Geometry: final body of the model. Coordinates: model frame, mm. Face numbers are marked on the shaded views. A direction names the side the tool comes from. Coordinates: 2 decimals unless noted, no trailing zeros. Write each loop counter-clockwise with the first axis right and the second up, starting at its lowest first coordinate (ties: lowest second). Pieces come first, ordered by that corner, then holes. Notation, with made-up numbers: (17.25, 42.5) - (67.25, 42.5) arc R34 cw to (67.25, 77.5) - close; hole circle Ø4 at (22.5, 34). An arc over 180 degrees is marked (long way). Answer as a JSON object with one key per item and string values. Group by question number.
Item 1: Mould query, pull axis Y, two halves, no side actions, for the marked faces 1, 2 and 3. Classes: pulls with the +Y half, pulls with the -Y half, needs draft (parallel to the pull), parting line crosses it, or undercut.
Item 2: Section B-B on x = 0. Return loops of the section in (y, z), and give its area (3 significant figures).
Item 3: Section A-A on y = 0. Return loops of the section in (x, z), and give its area (3 significant figures).
Item 4: Section D-D on y = 2.2. Return loops of the section in (x, z).
Item 5: Set-up query: the marked faces 4, 5 and 6. Return all of +Z, -Z, +X, -X, +Y, -Y with unobstructed straight access to the full face (end or side cutting, diameter ignored); none if empty.
Item 6: Line query: line 1 along Y through (x, z) = (0, -4.25); line 2 along X through (y, z) = (0, -4); line 3 along Y through (x, z) = (0, 0.5). Output: solid intervals per line, ascending. Write a range as from..to.
Item 7: Section C-C on z = 0. Return loops of the section in (x, y), and give its area (3 significant figures).
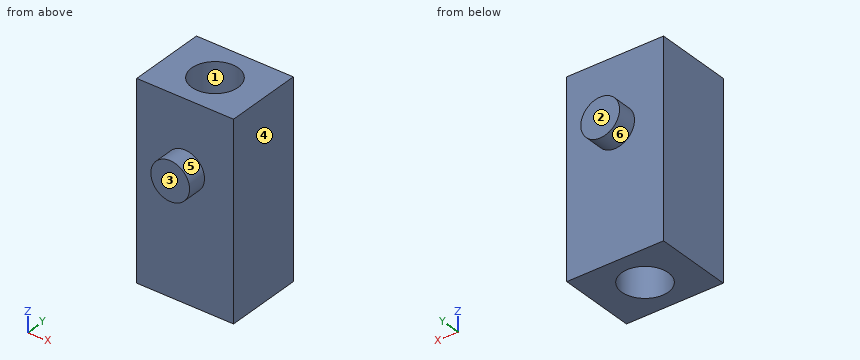
Autodesk Inventor part; units mm, degrees
ref_plane "YZ Plane" through (0, 0, 0) normal (1, 0, 0) x (0, 1, 0)
ref_plane "XZ Plane" through (0, 0, 0) normal (0, 1, 0) x (-1, 0, 0)
ref_plane "XY Plane" through (0, 0, 0) normal (0, 0, 1) x (1, 0, 0)
sketch "スケッチ1" plane through (0, 0, 0) normal (0, 1, 0) x (-1, 0, 0)
  line L0 (2.5, 3.5) -> (-2.5, 3.5)
  line L1 (-2.5, 3.5) -> (-2.5, -6.5)
  line L2 (-2.5, -6.5) -> (2.5, -6.5)
  line L3 (2.5, -6.5) -> (2.5, 3.5)
  point P0 (0, 0)
  point P1 (0, 3.5)
  dimension "d0" = 5
  dimension "d15" = 10
  dimension "d46" = 3.5
extrude "押し出し1" add sketch "スケッチ1" along normal mid plane 4
sketch "スケッチ2" plane through (0, 0, 0) normal (0, 1, 0) x (-1, 0, 0)
  circle A0 centre (0, 0) radius 1
  dimension "d3" = 2
extrude "押し出し2" add sketch "スケッチ2" along normal mid plane 6
sketch "スケッチ9" plane through (-2.5, 2, 3.5) normal (0, 0, 1) x (1, 0, 0)
  point P0 (2.5, -2)
  point P1 (2.5, -2)
hole "穴4" at (0, 0, 3.5) direction (0, 0, -1) diameter 2.4 end through all
properties part number "gear_connecotr1_V2" material "ABS プラスチック"
Checks:
{
 "1": {"face 1": "undercut", "face 2": "pulls with the +Y half", "face 3": "pulls with the -Y half"},
 "2": {"outline": "(-3, -1) - (-2, -1) - (-2, -6.5) - (-1.2, -6.5) - (-1.2, 3.5) - (-2, 3.5) - (-2, 1) - (-3, 1) - close; (1.2, -6.5) - (2, -6.5) - (2, -1) - (3, -1) - (3, 1) - (2, 1) - (2, 3.5) - (1.2, 3.5) - close", "area": "20.0 mm^2"},
 "3": {"outline": "(-2.5, -6.5) - (-1.2, -6.5) - (-1.2, 3.5) - (-2.5, 3.5) - close; (1.2, -6.5) - (2.5, -6.5) - (2.5, 3.5) - (1.2, 3.5) - close", "area": "26.0 mm^2"},
 "4": {"outline": "circle Ø2 at (0, 0)"},
 "5": {"face 4": "+Z, -Z, +X, +Y, -Y", "face 5": "-Y", "face 6": "+Y"},
 "6": {"line 1": "-2..-1.2, 1.2..2", "line 2": "-2.5..-1.2, 1.2..2.5", "line 3": "-3..-1.2, 1.2..3"},
 "7": {"outline": "(-2.5, -2) - (-1, -2) - (-1, -3) - (1, -3) - (1, -2) - (2.5, -2) - (2.5, 2) - (1, 2) - (1, 3) - (-1, 3) - (-1, 2) - (-2.5, 2) - close; hole circle Ø2.4 at (0, 0)", "area": "19.5 mm^2"}
}
